Can you work these out from the model? Positions are in its coordinate system, mm. A direction names the side the tool comes from. Give positions to 0.01 mm unless a question says otherwise; leave off trailing zeros. Loops run counter-clockwise (first coordinate to the right, second up) from the corner with the lowest first, then second, coordinate; pieces in that order, holes last.
from build123d import *

# Parameters (mm, degrees)
CUT_EXTRUDE_1_DEPTH      = 106.456152041
CUT_EXTRUDE_1_DEPTH_BACK = 106.456152041


with BuildPart() as part:
    # Эскиз1 → Повернуть1 (revolve)
    with BuildSketch(Plane.XY):
        with BuildLine():
            Line((0, 0), (0, 14.5))
            Line((0, 14.5), (-2.482050808, 15.933012702))
            ThreePointArc((-2.482050808, 15.933012702), (-2.602641285, 15.982962913), (-2.732050808, 16))
            Line((-2.732050808, 16), (-20.267949192, 16))
            ThreePointArc((-20.267949192, 16), (-20.397358715, 15.982962913), (-20.517949192, 15.933012702))
            Line((-20.517949192, 15.933012702), (-23, 14.5))
            Line((-23, 14.5), (-55, 14.5))
            Line((-55, 14.5), (-57.482050808, 15.933012702))
            ThreePointArc((-57.482050808, 15.933012702), (-57.602641285, 15.982962913), (-57.732050808, 16))
            Line((-57.732050808, 16), (-80.267949192, 16))
            ThreePointArc((-80.267949192, 16), (-80.397358715, 15.982962913), (-80.517949192, 15.933012702))
            Line((-80.517949192, 15.933012702), (-83, 14.5))
            Line((-83, 14.5), (-83, 7))
            Line((-83, 7), (-102.5, 7))
            Line((-102.5, 7), (-103, 6.5))
            Line((-103, 6.5), (-103, 0))
            Line((-103, 0), (0, 0))
        make_face()
    revolve(axis=Axis((0, 0, 0), (-1, 0, 0)))

    # Эскиз2 → Вырез-Вытянуть1 (cut, two sides: drawn at the far end of the back side and taken through both)
    with BuildSketch(Plane(origin=(0, 0, 0), x_dir=(1, 0, 0), z_dir=(0, 1, 0)).offset(-CUT_EXTRUDE_1_DEPTH_BACK)):
        with BuildLine():
            Line((-52, -8), (-26, -8))
            ThreePointArc((-26, -8), (-24.585786438, -7.414213562), (-24, -6))
            Line((-24, -6), (-24, 6))
            ThreePointArc((-24, 6), (-24.585786438, 7.414213562), (-26, 8))
            Line((-26, 8), (-52, 8))
            ThreePointArc((-52, 8), (-53.414213562, 7.414213562), (-54, 6))
            Line((-54, 6), (-54, -6))
            ThreePointArc((-54, -6), (-53.414213562, -7.414213562), (-52, -8))
        make_face()
    extrude(amount=CUT_EXTRUDE_1_DEPTH + CUT_EXTRUDE_1_DEPTH_BACK, mode=Mode.SUBTRACT)


solid = part.part
(1) Thinking about a two-plate mould opening in X: for faces 1 (the cylindrical face through (-11.62, -3.47, 15.62)), 2 (the flat face through (-83, -7, 3)), 3 (the flat face through (-54, 0, 0)), which applies, pulls with the +X half, pulls with the -X half, needs draft (parallel to the pull), parting line crosses it, or undercut?
Returned:
face 1: needs draft
face 2: pulls with the -X half
face 3: undercut
(2) Please list where these lines run through material, in increasing order: probe 1 along X at (y, z) = (7, -3.5); probe 2 along Z at (x, y) = (-49.5, 1); probe 3 along Y at (x, z) = (-62, -10.5).
Returned:
probe 1: x = -83 to -54, -24 to 0
probe 2: z = -14.47 to -8, 8 to 14.47
probe 3: y = -12.07 to 12.07
(3) Which directions (+Z, -Z, +X, -X, +Y, -Y) give clear straight access to the entire face, cutting with the end or side of a thin tool? Please do faces 4 (the cylindrical face through (-92.886, 6.466, 2.681)), 5 (the cylindrical face through (-39.22, -11.51, 8.82)), 6 (the flat face through (-24, 0, 0)).
Returned:
face 4: -X
face 5: none
face 6: +Y, -Y
(4) Suppose I cut it at B-B on x = -30. List the corners of the cut face in (y, z) for me, plus the area to 3 significant figures.
Returned:
outline: (-12.09, -8) arc R14.5 ccw to (12.09, -8) - close; (-12.09, 8) - (12.09, 8) arc R14.5 ccw to start
area: 221 mm2
(5) Suppose I cut it at C-C on x = -68. List the corners of the cut face in (y, z) for me, plus the area to 3 significant figures.
Returned:
outline: circle Ø32 at (0, 0)
area: 804 mm2
(6) Will these pins go through, and if not, where does the flat tip stop? P1, Ø1.5, axis at y = -12.5, z = -1, coming from the -X side; P2, Ø10, axis at x = -16.5, y = 11, coming from the -Z side; P3, Ø6, axis at x = -25.5, z = 1.5, coming from the +Y side.
Returned:
P1: stops at x = -83
P2: stops at z = -14.83
P3: stops at y = 14.73
